```python
from build123d import *

# Parameters (mm, degrees)
SKETCH1_R           = 95.25
BOSS_EXTRUDE1_DEPTH = 12.7
SKETCH2_R           = 54.356
CUT_EXTRUDE1_DEPTH  = 13.7
SKETCH3_R           = 64.135
CUT_EXTRUDE2_DEPTH  = 2.54
SKETCH4_R           = 2.794
CUT_EXTRUDE3_DEPTH  = 13.7
CIRPATTERN1_COUNT   = 12
SKETCH5_R           = 89.535
SKETCH5_R_2         = 85.09
CUT_EXTRUDE4_DEPTH  = 3.175


with BuildPart() as part:
    # Sketch1 → Boss-Extrude1 (new body)
    with BuildSketch(Plane(origin=(0, 0, 0), x_dir=(1, 0, 0), z_dir=(0, 1, 0))):
        Circle(SKETCH1_R)
    extrude(amount=BOSS_EXTRUDE1_DEPTH)

    # Sketch2 → Cut-Extrude1 (cut, through all)
    with BuildSketch(Plane(origin=(0, 12.7, 0), x_dir=(1, 0, 0), z_dir=(0, 1, 0))):
        Circle(SKETCH2_R)
    extrude(amount=-CUT_EXTRUDE1_DEPTH, mode=Mode.SUBTRACT)

    # Sketch3 → Cut-Extrude2 (cut)
    with BuildSketch(Plane(origin=(0, 12.7, 0), x_dir=(1, 0, 0), z_dir=(0, 1, 0))):
        Circle(SKETCH3_R)
    extrude(amount=-CUT_EXTRUDE2_DEPTH, mode=Mode.SUBTRACT)

    # Sketch4 → Cut-Extrude3 (cut, through all)
    with BuildSketch(Plane(origin=(0, 12.7, 0), x_dir=(1, 0, 0), z_dir=(0, 1, 0))):
        with Locations((0, 58.42)):
            Circle(SKETCH4_R)
    cut_extrude3 = extrude(amount=-CUT_EXTRUDE3_DEPTH, mode=Mode.SUBTRACT)

    # CirPattern1: Cut-Extrude3 ×12 about axis
    cirpattern1_axis = Axis((0, 0, 0), (0, 1, 0))
    for i in range(1, CIRPATTERN1_COUNT):
        add(cut_extrude3.rotate(cirpattern1_axis, i * 360 / CIRPATTERN1_COUNT), mode=Mode.SUBTRACT)

    # Sketch5 → Cut-Extrude4 (cut)
    with BuildSketch(Plane(origin=(0, 12.7, 0), x_dir=(1, 0, 0), z_dir=(0, 1, 0))):
        Circle(SKETCH5_R)
        Circle(SKETCH5_R_2, mode=Mode.SUBTRACT)
    extrude(amount=-CUT_EXTRUDE4_DEPTH, mode=Mode.SUBTRACT)


solid = part.part
```
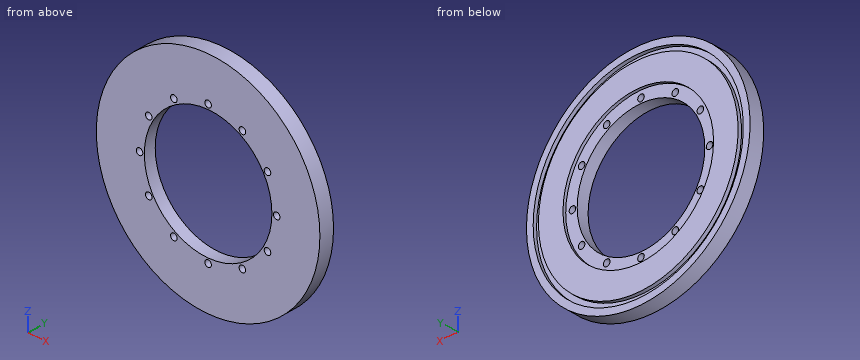
Could you check a few things on this model? Use its own coordinates, in mm. Round coordinates to 2 decimals unless told otherwise and drop trailing zeros. Loops run counter-clockwise (first coordinate to the right, second up) from the corner with the lowest first, then second, coordinate; pieces in that order, holes last. Notation, with made-up numbers: M 80.25,7.25 L 123.25,7.25 A15 ccw 123.25,11.25 Z; hole C -6,86 d7. An arc over 180 degrees is marked long. Answer as CSV lines item,"result".
1) For pin 1 Ø9 at (x, z) = (0, -58.42) entering from +Y; pin 2 Ø3 at (x, y) = (-25, 11) entering from -Z; pin 3 Ø4 at (y, z) = (8.5, 18) entering from +X, each with a flat end and sliding along its axis, tell me the tip position at first contact or that it passes through.
From the geometry:
pin 1,"y = 10.16"
pin 2,"z = -92.31"
pin 3,"x = 93.9"
2) Imagine slicing it at A-A on x = 36.5. List the corners of the cut face in (y, z) for me (3 decimals).
From the geometry:
outline,"M 0,-87.979 L 12.7,-87.979 L 12.7,-81.757 L 9.525,-81.757 L 9.525,-76.864 L 12.7,-76.864 L 12.7,-52.736 L 10.16,-52.736 L 10.16,-40.278 L 0,-40.278 Z; M 0,40.278 L 10.16,40.278 L 10.16,52.736 L 12.7,52.736 L 12.7,76.864 L 9.525,76.864 L 9.525,81.757 L 12.7,81.757 L 12.7,87.979 L 0,87.979 Z"
3) Imagine slicing it at B-B on z = 18.5. List the corners of the cut face in (x, y) for me (3 decimals).
From the geometry:
outline,"M -93.436,0 L -51.111,0 L -51.111,10.16 L -61.409,10.16 L -61.409,12.7 L -83.055,12.7 L -83.055,9.525 L -87.603,9.525 L -87.603,12.7 L -93.436,12.7 Z; M 51.111,0 L 93.436,0 L 93.436,12.7 L 87.603,12.7 L 87.603,9.525 L 83.055,9.525 L 83.055,12.7 L 61.409,12.7 L 61.409,10.16 L 51.111,10.16 Z"
4) Imagine slicing it at C-C on y = 7.5. Count the separate pieces of the cut face and the enclosed holes in it, and give its area (3 significant figures).
From the geometry:
separate pieces,"1"
enclosed holes,"13"
area,"18,900 mm^2"
5) If I drill on probe 1 along Z at (x, y) = (0, 2.75); probe 2 along Z at (x, y) = (0, 10.75) (3 decimals), over which ranges is the centre line in solid material (lowest first)?
From the geometry:
probe 1,"-95.25 to -61.21, -55.63 to -54.36, 54.36 to 55.63, 61.21 to 95.25"
probe 2,"-95.25 to -89.535, -85.09 to -64.135, 64.135 to 85.09, 89.535 to 95.25"
6) Imagine slicing it at D-D on z = -78.5. List the corners of the cut face in (x, y) for me (3 decimals), and give its area (3 significant figures).
From the geometry:
outline,"M -53.947,0 L 53.947,0 L 53.947,12.7 L 43.061,12.7 L 43.061,9.525 L 32.834,9.525 L 32.834,12.7 L -32.834,12.7 L -32.834,9.525 L -43.061,9.525 L -43.061,12.7 L -53.947,12.7 Z"
area,"1,310 mm^2"
